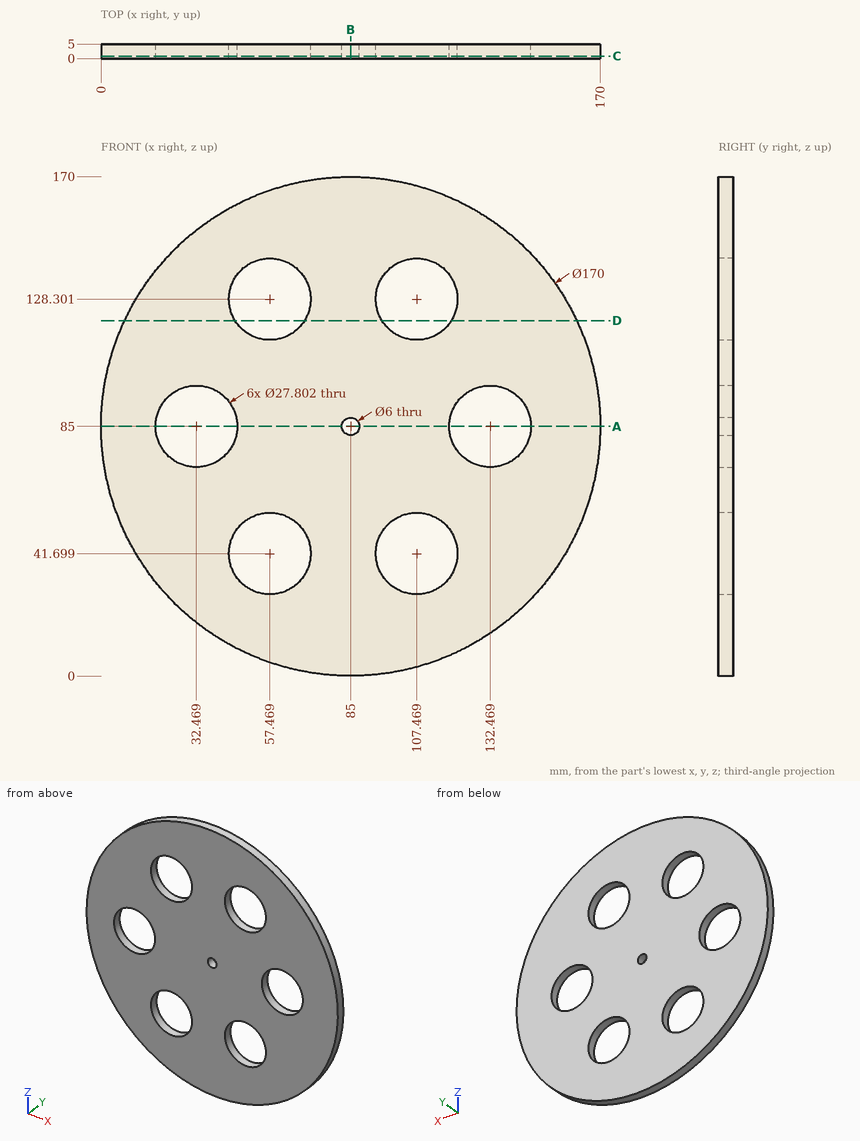
Part print with two shaded views. Sizes in mm from the minimum x, y, z corner. Give positions to 0.01 mm unless a question says otherwise; leave off trailing zeros. Order: outer loops, then holes, each group sorted by start corner. A loop starts at its lowest first (then second) coordinate and runs counter-clockwise, first axis right, second up. Notation, with made-up numbers: M -30,-30 L 26,-30 A24 ccw 26,1 Z; hole C 28,53.5 d6. An arc over 180 degrees is marked long. Use one line per item in the form item = value.
1) Drop a flat-ended pin along its axis: pin 1 (1.5 mm diameter, centred on x = 72, y = 3.5, fed in from -Z). Give the stop position or say it passes through.
Calculated:
pin_1 = 0.89
2) Probe probe 1 along X at (y, z) = (2.4, 85); probe 2 along X at (y, z) = (0.85, 40) (1 decimal); probe 3 along X at (y, z) = (3.95, 33.5) (1 decimal). List the from-to ranges inside material, lowest first.
Calculated:
probe_1 = 0 to 18.57, 46.37 to 82, 88 to 118.57, 146.37 to 170
probe_2 = 12.9 to 43.7, 71.3 to 93.7, 121.3 to 157.1
probe_3 = 17.4 to 46.2, 68.7 to 96.2, 118.7 to 152.6
3) Saw through at B-B (x = 85). Give the cut face in (y, z), plus the area to 3 significant figures.
Calculated:
outline = M 0,0 L 5,0 L 5,82 L 0,82 Z; M 0,88 L 5,88 L 5,170 L 0,170 Z
area = 820 mm2
4) Saw through at A-A (z = 85). Give the cut face in (x, y), plus the area to 3 significant figures.
Calculated:
outline = M 0,0 L 18.57,0 L 18.57,5 L 0,5 Z; M 46.37,0 L 82,0 L 82,5 L 46.37,5 Z; M 88,0 L 118.57,0 L 118.57,5 L 88,5 Z; M 146.37,0 L 170,0 L 170,5 L 146.37,5 Z
area = 542 mm2
5) Saw through at D-D (z = 121). Give the cut face in (x, y).
Calculated:
outline = M 8,0 L 45.64,0 L 45.64,5 L 8,5 Z; M 69.3,0 L 95.64,0 L 95.64,5 L 69.3,5 Z; M 119.3,0 L 162,0 L 162,5 L 119.3,5 Z
6) Saw through at C-C (y = 0.9). Give the cut face in (x, z), plus the area to 3 significant figures.
Calculated:
outline = C 85,85 d170; hole C 32.47,85 d27.8; hole C 57.47,41.7 d27.8; hole C 57.47,128.3 d27.8; hole C 85,85 d6; hole C 107.47,41.7 d27.8; hole C 107.47,128.3 d27.8; hole C 132.47,85 d27.8
area = 19,000 mm2
